```python
from build123d import *

# Parameters (mm, degrees)
SKIZZE1_R                       = 12.75
AUFSATZ_LINEAR_AUSTRAGEN1_DEPTH = 6.5
SKIZZE2_R                       = 2.25
SCHNITT_LINEAR_AUSTRAGEN1_DEPTH = 6.5


with BuildPart() as part:
    # Skizze1 → Aufsatz-Linear austragen1 (new, symmetric)
    with BuildSketch(Plane.XY):
        with Locations(Location((0, 0, 0), (0, 0, 180))):
            Circle(SKIZZE1_R)
    extrude(amount=AUFSATZ_LINEAR_AUSTRAGEN1_DEPTH, both=True)

    # Skizze2 → Schnitt-Linear austragen1 (cut, symmetric)
    with BuildSketch(Plane.XY):
        Circle(SKIZZE2_R)
    extrude(amount=SCHNITT_LINEAR_AUSTRAGEN1_DEPTH, both=True, mode=Mode.SUBTRACT)

    # Skizze3 → Schnitt-Rotation2 (revolve, cut)
    with BuildSketch(Plane(origin=(0, 0, 0), x_dir=(0, 0, -1), z_dir=(1, 0, 0))):
        with BuildLine():
            Line((-6.5, 10.968705484), (-6.5, 13.936393614))
            Line((-6.5, 13.936393614), (6.5, 13.936393614))
            Line((6.5, 13.936393614), (6.5, 10.968705484))
            ThreePointArc((6.5, 10.968705484), (0, 12.75), (-6.5, 10.968705484))
        make_face()
    revolve(axis=Axis((0, 0, 6.5), (0, 0, -1)), mode=Mode.SUBTRACT)


solid = part.part
```
Design review of the part built by this model. Coordinates are the model's own, in mm. Coordinates: 2 decimals unless noted, no trailing zeros. Write each loop counter-clockwise with the first axis right and the second up, starting at its lowest first coordinate (ties: lowest second). Pieces come first, ordered by that corner, then holes. Notation, with made-up numbers: M 5.5,56.25 L 39.5,56.25 A31 cw 39.5,84.25 Z; hole C -36.75,-24 d3. An arc over 180 degrees is marked long. Answer as a JSON object with one key per item and string values.
Item 1: Draft analysis for pull direction X (two halves, no side actions). For faces 1 (the flat face through (0, -3, -6.5)), 2 (the cylindrical face through (-0.29, 2.23, 0.09)), state which applies: pulls with the +X half, pulls with the -X half, needs draft (parallel to the pull), parting line crosses it, or undercut.
Outcome:
{"face 1": "needs draft", "face 2": "undercut"}
Item 2: Add section C-C, the plane z = -5.25. Give the boundary of the cut face in (x, y), and give its area (3 significant figures).
Outcome:
{"outline": "C 0,0 d23.24; hole C 0,0 d4.5", "area": "408 mm²"}
Item 3: Add section D-D, the plane x = -3.75. Give the boundary of the cut face in (y, z), and give its area (3 significant figures).
Outcome:
{"outline": "M -10.31,-6.5 L 10.31,-6.5 A12.19 ccw 10.31,6.5 L -10.31,6.5 A12.19 ccw Z", "area": "301 mm²"}
Item 4: Insertion check: pin 1 Ø3.5 at (x, y) = (0, 0) entering from -Z (3 decimals); pin 2 Ø6 at (y, z) = (4, -1) entering from +X; pin 3 Ø4 at (x, z) = (-8.5, -1.5) entering from -Y; pin 4 Ø6 at (x, z) = (1, -4) entering from -Y. Each pin has a flat end and moves straight along its axis. Give the tip position at first contact, or say it passes through.
Outcome:
{"pin 1": "through", "pin 2": "x = 12.7", "pin 3": "y = -10.89", "pin 4": "y = -12.7"}
Item 5: Add section A-A, the plane x = 0. Give the boundary of the cut face in (y, z), and give its area (3 significant figures).
Outcome:
{"outline": "M -10.97,-6.5 L -2.25,-6.5 L -2.25,6.5 L -10.97,6.5 A12.75 ccw Z; M 2.25,-6.5 L 10.97,-6.5 A12.75 ccw 10.97,6.5 L 2.25,6.5 Z", "area": "258 mm²"}
Item 6: Wall thickness on probe 1 along Y at (x, z) = (0, 0); probe 2 along Y at (x, z) = (0, -2.75); probe 3 along X at (y, z) = (-1.75, 3.5): over which ranges is each line inside the solid? List them lowest first.
Outcome:
{"probe 1": "-12.75 to -2.25, 2.25 to 12.75", "probe 2": "-12.45 to -2.25, 2.25 to 12.45", "probe 3": "-12.13 to -1.41, 1.41 to 12.13"}
